Geometry: final body of the model. Coordinates: model frame, mm. Face numbers are marked on the shaded views. A direction names the side the tool comes from. Round coordinates to 2 decimals unless told otherwise and drop trailing zeros. Loops run counter-clockwise (first coordinate to the right, second up) from the corner with the lowest first, then second, coordinate; pieces in that order, holes last. Notation, with made-up numbers: (39.25, -2.75) -> (68.25, -2.75) arc R23 ccw to (68.25, 15.25) -> close; hole circle Ø3 at (65, -30). An arc over 180 degrees is marked (long way). Answer in a Markdown table with one row per item.
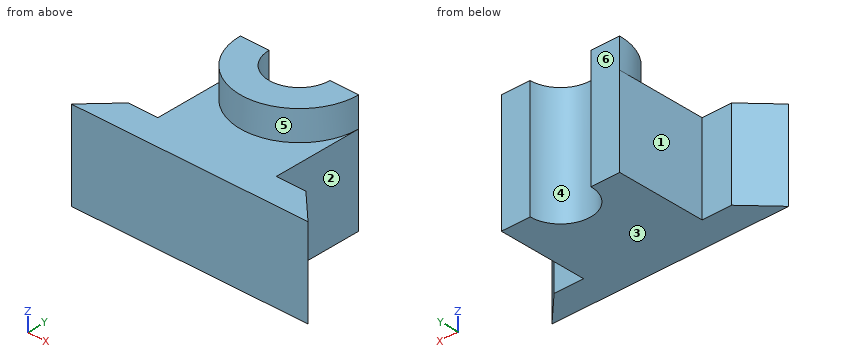
```python
from build123d import *

# Parameters (mm, degrees)
BOSS_EXTRUDE1_DEPTH = 762
BOSS_EXTRUDE2_DEPTH = 1016


with BuildPart() as part:
    # Sketch1 → Boss-Extrude1 (new body)
    with BuildSketch(Plane.XY):
        with BuildLine():
            Line((508, 0), (508, -762))
            Line((508, -762), (762, -762))
            Line((762, -762), (1016, -1016))
            Line((1016, -1016), (-1016, -1016))
            Line((-1016, -1016), (-762, -762))
            Line((-762, -762), (-508, -762))
            Line((-508, -762), (-508, 0))
            ThreePointArc((-508, 0), (0, -508), (508, 0))
        make_face()
    extrude(amount=BOSS_EXTRUDE1_DEPTH)

    # Sketch1_3 → Boss-Extrude2 (add)
    with BuildSketch(Plane.XY):
        with BuildLine():
            Line((-508, 0), (-260.853189007, 0))
            ThreePointArc((-260.853189007, 0), (0, -260.853189007), (260.853189007, 0))
            Line((260.853189007, 0), (508, 0))
            ThreePointArc((508, 0), (0, -508), (-508, 0))
        make_face()
    extrude(amount=BOSS_EXTRUDE2_DEPTH)


solid = part.part
```
Item 1: Line query: probe 1 along Z at (x, y) = (447.5, -435); probe 2 along X at (y, z) = (-519, 345.5); probe 3 along Y at (x, z) = (619.5, 201). Output: solid intervals per line, ascending. Write a range as [from, to].
Answer:
| item | result |
|---|---|
| probe 1 | z = [0, 762] |
| probe 2 | x = [-508, 508] |
| probe 3 | y = [-1016, -762] |
Item 2: Reachability of the marked faces 1, 2 and 3 from +Z, -Z, +X, -X, +Y, -Y: full face, straight path, thin tool, end or side. Return the list, or none.
Answer:
| item | result |
|---|---|
| face 1 | +Z, -Z, -X, +Y |
| face 2 | +Z, -Z, +X, +Y |
| face 3 | -Z, +X, -X, +Y, -Y |
Item 3: Draft query along X for the marked faces 4, 5 and 6. Return one class per face: pulls with the +X half, pulls with the -X half, needs draft (parallel to the pull), parting line crosses it, or undercut.
Answer:
| item | result |
|---|---|
| face 4 | undercut |
| face 5 | parting line crosses it |
| face 6 | needs draft |
Item 4: Cut plane D-D (y = -334). Output: boundary loops of the cut face in (x, z).
Answer:
| item | result |
|---|---|
| outline | (-508, 0) -> (508, 0) -> (508, 762) -> (382.76, 762) -> (382.76, 1016) -> (-382.76, 1016) -> (-382.76, 762) -> (-508, 762) -> close |
Item 5: Cut plane A-A (y = -158.5). Output: boundary loops of the cut face in (x, z).
Answer:
| item | result |
|---|---|
| outline | (-508, 0) -> (-207.18, 0) -> (-207.18, 1016) -> (-482.64, 1016) -> (-482.64, 762) -> (-508, 762) -> close; (207.18, 0) -> (508, 0) -> (508, 762) -> (482.64, 762) -> (482.64, 1016) -> (207.18, 1016) -> close |
Item 6: Cut plane B-B (z = 144). Output: boundary loops of the cut face in (x, y), then the cut area to 3 significant figures.
Answer:
| item | result |
|---|---|
| outline | (-1016, -1016) -> (1016, -1016) -> (762, -762) -> (508, -762) -> (508, 0) -> (260.85, 0) arc R260.85 cw to (-260.85, 0) -> (-508, 0) -> (-508, -762) -> (-762, -762) -> close |
| area | 1,120,000 mm² |
Item 7: Cut plane C-C (x = 0). Output: boundary loops of the cut face in (y, z), then the cut area to 3 significant figures.
Answer:
| item | result |
|---|---|
| outline | (-1016, 0) -> (-260.85, 0) -> (-260.85, 1016) -> (-508, 1016) -> (-508, 762) -> (-1016, 762) -> close |
| area | 638,000 mm² |
Item 8: Pin query (flat end, axial travel): pin 1 Ø8 at (y, z) = (-246, 117.5) entering from +X; pin 2 Ø8 at (y, z) = (-244, 481.5) entering from -X; pin 3 Ø1 at (y, z) = (-444.5, 785) entering from +X. Return the tip coordinate at first contact, or that it passes through.
Answer:
| item | result |
|---|---|
| pin 1 | stops at x = 508 |
| pin 2 | stops at x = -508 |
| pin 3 | stops at x = 246.84 |
